Geometry: final body of the model. Coordinates: model frame, mm. Face numbers are marked on the shaded views. A direction names the side the tool comes from. Coordinates: 2 decimals unless noted, no trailing zeros. Order: outer loops, then holes, each group sorted by start corner. A loop starts at its lowest first (then second) coordinate and runs counter-clockwise, first axis right, second up. Notation, with made-up numbers: M -22,71 L 12,71 A14 cw 12,82 Z; hole C 80.25,46.25 d10. An arc over 180 degrees is marked long. Use CSV: the item, a comma, the result in double quotes. Start each with the question number.
1. Section query D-D on y = 0. Return the cut outline in (x, z).
2. Section query B-B on x = 15.5. Return the cut outline in (y, z), and give its area (3 significant figures).
3. Material intervals for line 1 (Y direction, x = -22, z = 6.25); line 2 (X direction, y = 1, z = 12); line 3 (Y direction, x = 50.5, z = 5), sorted ascending.
4. Set-up query: the marked faces 1 and 2. Return all of +Z, -Z, +X, -X, +Y, -Y with unobstructed straight access to the full face (end or side cutting, diameter ignored); none if empty.
5. Section query A-A on y = -12.5. Return the cut outline in (x, z), and give its area (3 significant figures).
6. Section query C-C on z = 3.5. Return the cut outline in (x, y), and give its area (3 significant figures).
7. Pull-direction query (Y, two-part tool) for the marked faces 3, 4, 5 and 6; classes: pulls with the +Y half, pulls with the -Y half, needs draft (parallel to the pull), parting line crosses it, or undercut.
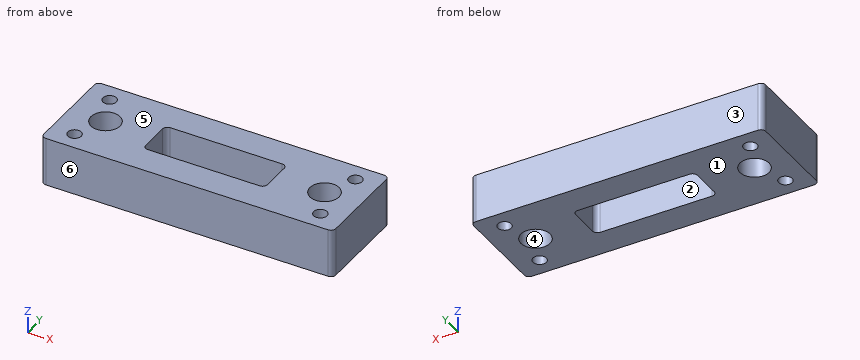
from build123d import *

# Parameters (mm, degrees)
SKETCH_1_W          = 120
SKETCH_1_H          = 40
EXTRUDE_1_DEPTH     = 20
SKETCH_2_R          = 6
SKETCH_2_R_2        = 2.75
CUT_EXTRUDE_1_DEPTH = 20
FILLET_1_R          = 2
SKETCH_3_W          = 50
SKETCH_3_H          = 16
CUT_EXTRUDE_2_DEPTH = 67.332495807
FILLET_2_R          = 2


with BuildPart() as part:
    # 草图1 → 凸台-拉伸1 (new body)
    with BuildSketch(Plane.XY):
        Rectangle(SKETCH_1_W, SKETCH_1_H)
    extrude(amount=EXTRUDE_1_DEPTH)

    # 草图2 → 切除-拉伸1 (cut)
    with BuildSketch(Plane.XY.offset(20)):
        with Locations((45, 0)):
            Circle(SKETCH_2_R)
        with Locations((50.5, 12.5)):
            Circle(SKETCH_2_R_2)
        with Locations(Location((50.5, -12.5, 0), (0, 0, 180))):
            Circle(SKETCH_2_R_2)
        with Locations((-50.5, -12.5)):
            Circle(SKETCH_2_R_2)
        with Locations(Location((-50.5, 12.5, 0), (0, 0, 180))):
            Circle(SKETCH_2_R_2)
        with Locations(Location((-45, 0, 0), (0, 0, 180))):
            Circle(SKETCH_2_R)
    extrude(amount=-CUT_EXTRUDE_1_DEPTH, mode=Mode.SUBTRACT)

    # 圆角1
    fillet_1_edges = [part.edges().sort_by_distance(p)[0] for p in [
        (-60, 20, 10),
        (60, 20, 10),
        (60, -20, 10),
        (-60, -20, 10),
    ]]
    fillet(fillet_1_edges, radius=FILLET_1_R)

    # 草图3 → 切除-拉伸2 (cut, through all)
    with BuildSketch(Plane.XY.offset(20)):
        Rectangle(SKETCH_3_W, SKETCH_3_H)
    extrude(amount=-CUT_EXTRUDE_2_DEPTH, mode=Mode.SUBTRACT)

    # 圆角2
    fillet_2_edges = [part.edges().sort_by_distance(p)[0] for p in [
        (-25, -8, 10),
        (-25, 8, 10),
        (25, 8, 10),
        (25, -8, 10),
    ]]
    fillet(fillet_2_edges, radius=FILLET_2_R)


solid = part.part
Results list:
1,outline,"M -60,0 L -51,0 L -51,20 L -60,20 Z; M -39,0 L -25,0 L -25,20 L -39,20 Z; M 25,0 L 39,0 L 39,20 L 25,20 Z; M 51,0 L 60,0 L 60,20 L 51,20 Z"
2,outline,"M -20,0 L -8,0 L -8,20 L -20,20 Z; M 8,0 L 20,0 L 20,20 L 8,20 Z"
2,area,"480 mm²"
3,line 1,"y = -20 to -8, 8 to 20"
3,line 2,"x = -60 to -50.92, -39.08 to -25, 25 to 39.08, 50.92 to 60"
3,line 3,"y = -20 to -15.25, -9.75 to -2.4, 2.4 to 9.75, 15.25 to 20"
4,face 1,"-Z, +X, -X, +Y, -Y"
4,face 2,"+Z, -Z"
5,outline,"M -60,0 L -53.25,0 L -53.25,20 L -60,20 Z; M -47.75,0 L 47.75,0 L 47.75,20 L -47.75,20 Z; M 53.25,0 L 60,0 L 60,20 L 53.25,20 Z"
5,area,"2,180 mm²"
6,outline,"M -60,-18 A2 ccw -58,-20 L 58,-20 A2 ccw 60,-18 L 60,18 A2 ccw 58,20 L -58,20 A2 ccw -60,18 Z; hole C -50.5,-12.5 d5.5; hole C -50.5,12.5 d5.5; hole C -45,0 d12; hole M -25,-6 A2 ccw -23,-8 L 23,-8 A2 ccw 25,-6 L 25,6 A2 ccw 23,8 L -23,8 A2 ccw -25,6 Z; hole C 45,0 d12; hole C 50.5,-12.5 d5.5; hole C 50.5,12.5 d5.5"
6,area,"3,680 mm²"
7,face 3,"pulls with the +Y half"
7,face 4,"undercut"
7,face 5,"needs draft"
7,face 6,"pulls with the -Y half"
